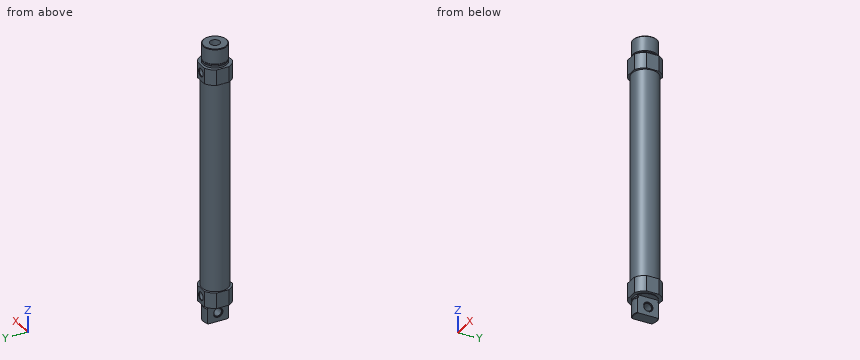
Autodesk Inventor part; units mm, degrees
ref_plane "FDT_FRONT_XY" through (0, 0, -30.1) normal (0, 0, -1) x (1, 0, 0)
ref_plane "FDT_FRONT_YZ" through (0, 0, -30.1) normal (1, 0, 0) x (0, -1, 0)
ref_plane "FDT_FRONT_ZX" through (0, 0, -30.1) normal (0, -1, 0) x (0, 0, -1)
sketch "Sketch_12" plane through (0, 0, 0) normal (1, 0, 0) x (0, 1, 0)
  line L0 (0, -444.6) -> (0, 0)
  line L1 (0, 0) -> (18.08, 0)
  line L2 (18.08, 0) -> (19, -0.92)
  line L3 (19, -0.92) -> (19, -23.95)
  line L4 (19, -23.95) -> (18.0843, -24.8657)
  arc A0 (18.0843, -24.8657) -> (17.85, -25.4314) centre (18.65, -25.4314) ccw
  line L5 (17.85, -25.4314) -> (17.85, -26.2)
  arc A1 (17.85, -26.2) -> (18.65, -27) centre (18.65, -26.2) ccw
  line L6 (18.65, -27) -> (19, -27)
  line L7 (19, -27) -> (19, -30.1)
  line L8 (19, -30.1) -> (24.5, -30.1)
  line L9 (24.5, -30.1) -> (24.5, -55.05)
  line L10 (24.5, -55.05) -> (20.8, -55.05)
  line L11 (20.8, -55.05) -> (20.8, -389.55)
  line L12 (20.8, -389.55) -> (24.5, -389.55)
  line L13 (24.5, -389.55) -> (24.5, -414.5)
  line L14 (24.5, -414.5) -> (19, -414.5)
  line L15 (19, -414.5) -> (19, -417.6)
  line L16 (19, -417.6) -> (18.65, -417.6)
  arc A2 (18.65, -417.6) -> (17.85, -418.4) centre (18.65, -418.4) ccw
  line L17 (17.85, -418.4) -> (17.85, -419.1686)
  arc A3 (17.85, -419.1686) -> (18.0843, -419.7343) centre (18.65, -419.1686) ccw
  line L18 (18.0843, -419.7343) -> (19, -420.65)
  line L19 (19, -420.65) -> (19, -443.68)
  line L20 (19, -443.68) -> (18.08, -444.6)
  line L21 (18.08, -444.6) -> (0, -444.6)
  line L22 (0, -444.6) -> (0, 0)
revolve "Revolution1" add sketch "Sketch_12" angle 360 about axis through (0, 0, -444.6) along (0, 0, -1)
thread "Thread1"
thread "Thread2"
sketch "Sketch_1" plane through (0, 0, 0) normal (0, 0, 1) x (1, 0, 0)
  line L0 (-45, 45) -> (-45, -45)
  line L1 (-45, -45) -> (45, -45)
  line L2 (45, -45) -> (45, 45)
  line L3 (45, 45) -> (-45, 45)
  line L4 (-22.5, 22.5) -> (-22.5, -22.5)
  line L5 (-22.5, -22.5) -> (22.5, -22.5)
  line L6 (22.5, -22.5) -> (22.5, 22.5)
  line L7 (22.5, 22.5) -> (-22.5, 22.5)
extrude "Extrusion1" cut sketch "Sketch_1" against normal blind 453.6
sketch "Sketch_124" plane through (0, 0, 0) normal (0, 1, 0) x (-1, 0, 0)
  line L0 (46, -415.6) -> (9, -415.6)
  line L1 (9, -415.6) -> (9, -444.6)
  line L2 (9, -444.6) -> (-9, -444.6)
  line L3 (-9, -444.6) -> (-9, -415.6)
  line L4 (-9, -415.6) -> (-46, -415.6)
  line L5 (-46, -415.6) -> (-46, -449.6)
  line L6 (-46, -449.6) -> (46, -449.6)
  line L7 (46, -449.6) -> (46, -415.6)
extrude "Extrusion2" cut sketch "Sketch_124" along normal mid plane 46
sketch "Sketch_3" plane through (0, 0, -430.6) normal (0, 0, 1) x (1, 0, 0)
  line L0 (9, 0) -> (-9, 0)
  line L1 (-9, 0) -> (-9, 7.5774)
  line L2 (-9, 7.5774) -> (-8, 7)
  line L3 (-8, 7) -> (-7.5, 7)
  line L4 (-7.5, 7) -> (-7.5, 6)
  line L5 (-7.5, 6) -> (7.5, 6)
  line L6 (7.5, 6) -> (7.5, 7)
  line L7 (7.5, 7) -> (8, 7)
  line L8 (8, 7) -> (9, 7.5774)
  line L9 (9, 7.5774) -> (9, 0)
  line L10 (9, 0) -> (-9, 0)
revolve "Revolution2" cut sketch "Sketch_3" angle 360 about axis through (9, 0, -430.6) along (1, 0, 0)
sketch "Sketch5" plane through (-9.6954, 22.5, -30.1) normal (0, 1, 0) x (1, 0, 0)
  point P0 (9.6954, 12)
hole "Hole1" at (0, 22.5, -42.1) direction (0, -1, 0) diameter 11.445 depth 22.5 countersink diameter 13.157 countersink angle 90
sketch "Sketch6" plane through (-9.6954, 22.5, -389.55) normal (0, 1, 0) x (1, 0, 0)
  point P0 (9.6954, 12.95)
hole "Hole2" at (0, 22.5, -402.5) direction (0, -1, 0) diameter 11.445 depth 10.5 tip angle 120 countersink diameter 13.157 countersink angle 90
sketch "Sketch_129" plane through (0, 0, 0) normal (1, 0, 0) x (0, 1, 0)
  line L0 (0, -377) -> (0, 9)
  line L1 (0, 9) -> (8, 9)
  line L2 (8, 9) -> (8, -67)
  line L3 (8, -67) -> (20, -67)
  line L4 (20, -67) -> (20, -377)
  line L5 (20, -377) -> (0, -377)
  line L6 (0, -377) -> (0, 9)
revolve "Revolution3" cut sketch "Sketch_129" angle 360 about axis through (0, 0, -377) along (0, 0, -1)
ref_plane "FDT_FRONT_XY" through (0, 0, -30.1) normal (0, 0, -1) x (1, 0, 0)
ref_plane "FDT_FRONT_YZ" through (0, 0, -30.1) normal (1, 0, 0) x (0, -1, 0)
ref_plane "FDT_FRONT_ZX" through (0, 0, -30.1) normal (0, -1, 0) x (0, 0, -1)
ref_plane "FDT_QSFRONT_XY" through (0, 22.5, -42.1) normal (0, 1, 0) x (0, 0, 1)
ref_plane "FDT_QSFRONT_YZ" through (0, 22.5, -42.1) normal (0, 0, 1) x (1, 0, 0)
ref_plane "FDT_QSFRONT_ZX" through (0, 22.5, -42.1) normal (1, 0, 0) x (0, 1, 0)
ref_plane "FDT_QSREAR_XY" through (0, 22.5, -402.5) normal (0, 1, 0) x (0, 0, 1)
ref_plane "FDT_QSREAR_YZ" through (0, 22.5, -402.5) normal (0, 0, 1) x (1, 0, 0)
ref_plane "FDT_QSREAR_ZX" through (0, 22.5, -402.5) normal (1, 0, 0) x (0, 1, 0)
ref_plane "FDT_REAR_XY" through (0, 0, -414.5) normal (0, 0, 1) x (1, 0, 0)
ref_plane "FDT_REAR_YZ" through (0, 0, -414.5) normal (1, 0, 0) x (0, 1, 0)
ref_plane "FDT_REAR_ZX" through (0, 0, -414.5) normal (0, 1, 0) x (0, 0, 1)
ref_plane "FDT_SMBR1_XY" through (0, 0, -64.5) normal (0, 0, 1) x (-1, 0, 0)
ref_plane "FDT_SMBR1_YZ" through (0, 0, -64.5) normal (-1, 0, 0) x (0, -1, 0)
ref_plane "FDT_SMBR1_ZX" through (0, 0, -64.5) normal (0, -1, 0) x (0, 0, 1)
ref_plane "FDT_SMBR2_XY" through (0, 0, -380.1) normal (0, 0, 1) x (-1, 0, 0)
ref_plane "FDT_SMBR2_YZ" through (0, 0, -380.1) normal (-1, 0, 0) x (0, -1, 0)
ref_plane "FDT_SMBR2_ZX" through (0, 0, -380.1) normal (0, -1, 0) x (0, 0, 1)
ref_plane "FDT_SWIVELAXIS_XY" through (0, 0, -430.6) normal (1, 0, 0) x (0, 0, -1)
ref_plane "FDT_SWIVELAXIS_YZ" through (0, 0, -430.6) normal (0, 0, -1) x (0, 1, 0)
ref_plane "FDT_SWIVELAXIS_ZX" through (0, 0, -430.6) normal (0, 1, 0) x (1, 0, 0)
ref_plane "NUT_XY" through (0, 0, -8.5) normal (0, 0, -1) x (1, 0, 0)
ref_plane "NUT_YZ" through (0, 0, -8.5) normal (1, 0, 0) x (0, -1, 0)
ref_plane "NUT_ZX" through (0, 0, -8.5) normal (0, -1, 0) x (0, 0, -1)
ref_plane "ZR_XY" through (0, 0, 0) normal (0, 0, -1) x (-1, 0, 0)
ref_plane "ZR_YZ" through (0, 0, 0) normal (-1, 0, 0) x (0, 1, 0)
ref_plane "ZR_ZX" through (0, 0, 0) normal (0, 1, 0) x (0, 0, -1)
ref_plane "ZYL_XY" through (0, 0, -30.1) normal (0, 0, -1) x (1, 0, 0)
ref_plane "ZYL_YZ" through (0, 0, -30.1) normal (1, 0, 0) x (0, -1, 0)
ref_plane "ZYL_ZX" through (0, 0, -30.1) normal (0, -1, 0) x (0, 0, -1)
properties part number "193993 DSNU-40-300-P---(A----0-ZR)"
Source: CAD feature listing. Evaluate the final solid. Frame: model axes, mm. Give positions to 0.01 mm unless a question says otherwise; leave off trailing zeros. Order: outer loops, then holes, each group sorted by start corner. A loop starts at its lowest first (then second) coordinate and runs counter-clockwise, first axis right, second up.
(1) Material intervals for line 1 along Z through (x, y) = (0, 17.25); line 2 along Z through (x, y) = (12, -8.5); line 3 along Z through (x, y) = (-17, -16), sorted ascending.
(2) Contact query for flat-ended pins moving along their axis: P1, Ø7, axis at y = 3, z = -429, coming from the +X side; P2, Ø10, axis at x = -15, y = 0.5, coming from the +Z side; P3, Ø4, axis at x = -16, y = -12, coming from the -Z side; P4, Ø16, axis at y = 0, z = -430.6, coming from the +X side. Output: stop coordinate, or through.
(3) Section query B-B (z = -42.1). Return the cut outline in (x, y).
(4) Section query A-A (z = -430.6). Return the cut outline in (x, y).
Outcome:
1. line 1: z = -444.6 to -408.22, -396.78 to -377, -67 to -47.82, -36.38 to 0
1. line 2: z = -415.6 to -377, -67 to 0
1. line 3: z = -414.5 to -389.55, -55.05 to -30.1
2. P1: stops at x = 7.5
2. P2: stops at z = 0
2. P3: stops at z = -415.6
2. P4: stops at x = 9
3. outline: (-22.5, -9.7) arc R24.5 ccw to (-9.7, -22.5) - (9.7, -22.5) arc R24.5 ccw to (22.5, -9.7) - (22.5, 9.7) arc R24.5 ccw to (9.7, 22.5) - (6.58, 22.5) - (5.72, 21.64) - (5.72, 5.59) arc R8 cw (long way) to (-5.72, 5.59) - (-5.72, 21.64) - (-6.58, 22.5) - (-9.7, 22.5) arc R24.5 ccw to (-22.5, 9.7) - close
4. outline: (-9, -16.73) arc R19 ccw to (9, -16.73) - (9, -7.58) - (8, -7) - (7.5, -7) - (7.5, -6) - (-7.5, -6) - (-7.5, -7) - (-8, -7) - (-9, -7.58) - close; (-9, 7.58) - (-8, 7) - (-7.5, 7) - (-7.5, 6) - (7.5, 6) - (7.5, 7) - (8, 7) - (9, 7.58) - (9, 16.73) arc R19 ccw to (-9, 16.73) - close
